Design review of the part built by this model. Coordinates are the model's own, in mm. A direction names the side the tool comes from. Give positions to 0.01 mm unless a question says otherwise; leave off trailing zeros. Order: outer loops, then holes, each group sorted by start corner. A loop starts at its lowest first (then second) coordinate and runs counter-clockwise, first axis right, second up.
```python
from build123d import *

# Parameters (mm, degrees)
ESQUISSE2_R                         = 1.35
BOSS_EXTRU_2_DEPTH                  = 6
BOSS_EXTRU_3_START                  = -6
ESQUISSE3_R                         = 1.35
BOSS_EXTRU_3_DEPTH                  = 6
ENL_V_MAT_EXTRU_1_REACH             = 49.73
ESQUISSE4_W                         = 8
ESQUISSE4_H                         = 4
ENL_V_MAT_EXTRU_1_DIRECTION_2_REACH = 49.73
CONG_1_R                            = 5


with BuildPart() as part:
    # Esquisse1 → Révolution1 (revolve)
    with BuildSketch(Plane.XY, mode=Mode.PRIVATE) as r_volution1_sk:
        Polygon((-6.05, 0), (-6.05, 4), (-3.85, 4), (-3.25, 4.6), (-3.25, 25.8), (-3.85, 26.4), (-6.05, 26.4), (-6.05, 30.4), (-8, 30.4), (-8, 24.4), (-5, 21.4), (-5, 9), (-8, 6), (-8, 0), align=None)
    revolve(r_volution1_sk.sketch.rotate(Axis((0, -1.144220684, 0), (0, 1, 0)), 270), axis=Axis((0, -1.144220684, 0), (0, 1, 0)))

    # Esquisse2 → Boss.-Extru.2 (add)
    with BuildSketch(Plane(origin=(0, 0, 0), x_dir=(1, 0, 0), z_dir=(0, 1, 0))):
        with BuildLine():
            Line((-7.878088106, -1.391304348), (-3.939044053, -23.695652174))
            ThreePointArc((-3.939044053, -23.695652174), (0, -27), (3.939044053, -23.695652174))
            Line((3.939044053, -23.695652174), (7.878088106, -1.391304348))
            ThreePointArc((7.878088106, -1.391304348), (0, -8), (-7.878088106, -1.391304348))
        make_face()
        with Locations(Location((0, -23, 0), (0, 0, 270))):
            Circle(ESQUISSE2_R, mode=Mode.SUBTRACT)
    extrude(amount=BOSS_EXTRU_2_DEPTH)

    # Esquisse3 → Boss.-Extru.3 (add)
    with BuildSketch(Plane(origin=(0, 30.4, 0), x_dir=(1, 0, 0), z_dir=(0, 1, 0)).offset(BOSS_EXTRU_3_START)):
        with BuildLine():
            Line((-21.761904762, -3.926767262), (-1.523809524, -7.853534525))
            ThreePointArc((-1.523809524, -7.853534525), (-8, 0), (-1.523809524, 7.853534525))
            Line((-1.523809524, 7.853534525), (-21.761904762, 3.926767262))
            ThreePointArc((-21.761904762, 3.926767262), (-25, 0), (-21.761904762, -3.926767262))
        make_face()
        with Locations(Location((-21, 0, 0), (0, 0, 270))):
            Circle(ESQUISSE3_R, mode=Mode.SUBTRACT)
    extrude(amount=BOSS_EXTRU_3_DEPTH)

    # Enlèv. mat.-Extru.1: up to this plane
    enl_v_mat_extru_1_end = Plane(origin=(-21.761904762, 24.4, -3.926767262), z_dir=(-0.19047619047618092, 0, -0.9816918156232545))
    # Esquisse4 → Enlèv. mat.-Extru.1 (cut, up to the surface)
    with BuildSketch(Plane.XY, mode=Mode.PRIVATE) as enl_v_mat_extru_1_sk1:
        with Locations((-21, 28.4)):
            Rectangle(ESQUISSE4_W, ESQUISSE4_H)
    enl_v_mat_extru_1_tool1 = split(extrude(enl_v_mat_extru_1_sk1.sketch, amount=-ENL_V_MAT_EXTRU_1_REACH, mode=Mode.PRIVATE), bisect_by=enl_v_mat_extru_1_end, keep=Keep.BOTH, mode=Mode.PRIVATE)
    add(enl_v_mat_extru_1_tool1.solids().sort_by_distance((-21, 28.4, 0))[0], mode=Mode.SUBTRACT)

    # Enlèv. mat.-Extru.1 direction 2: up to this plane
    enl_v_mat_extru_1_direction_2_end = Plane(origin=(-21.761904762, 24.4, 3.926767262), z_dir=(-0.19047619047620132, 0, 0.9816918156232504))
    # Esquisse4 → Enlèv. mat.-Extru.1 direction 2 (cut, up to the surface)
    with BuildSketch(Plane.XY, mode=Mode.PRIVATE) as enl_v_mat_extru_1_direction_2_sk1:
        with Locations((-21, 28.4)):
            Rectangle(ESQUISSE4_W, ESQUISSE4_H)
    enl_v_mat_extru_1_direction_2_tool1 = split(extrude(enl_v_mat_extru_1_direction_2_sk1.sketch, amount=ENL_V_MAT_EXTRU_1_DIRECTION_2_REACH, mode=Mode.PRIVATE), bisect_by=enl_v_mat_extru_1_direction_2_end, keep=Keep.BOTH, mode=Mode.PRIVATE)
    add(enl_v_mat_extru_1_direction_2_tool1.solids().sort_by_distance((-21, 28.4, 0))[0], mode=Mode.SUBTRACT)

    # Congé1
    cong_1_edges = [part.edges().sort_by_distance(p)[0] for p in [
        (-17, 28.4, -4.850712501),
        (-17, 28.4, 4.850712501),
    ]]
    fillet(cong_1_edges, radius=CONG_1_R)


solid = part.part
```
1. For line 1 along X through (y, z) = (25.7, 0); line 2 along X through (y, z) = (11, 0); line 3 along X through (y, z) = (2.05, 0), list the stretches that pass through material, from the lowest coordinate up.
Recorded:
line 1: x = -25 to -22.35, -19.65 to -3.25, 3.25 to 8
line 2: x = -5 to -3.25, 3.25 to 5
line 3: x = -8 to -6.05, 6.05 to 8
2. For pin 1 (3.5 mm diameter, centred on x = -21, z = 0, fed in from +Y); pin 2 (6 mm diameter, centred on x = -8.5, y = 19, fed in from +Z); pin 3 (1.6 mm diameter, centred on y = 28, z = 0, fed in from -X); pin 4 (6 mm diameter, centred on y = 6, z = 17.5, fed in from +X), all flat-tipped, find the tip position at first contact; note any pin that passes through.
Recorded:
pin 1: stops at y = 26.4
pin 2: passes through
pin 3: stops at x = -17
pin 4: stops at x = 5.56
3. Take a section at A-A (x = 0). State how many separate pieces and enclosed holes the cut face has, then the cut area to 3 significant figures.
Recorded:
separate pieces: 3
enclosed holes: 0
area: 249 mm2
4. Machinability: for faces 1 (the face through (-15.89, 28.43, -3.87)), 2 (the face through (-15.89, 28.43, 3.87)), 3 (the face through (1, 4, -4)), which of the approach directions +Z, -Z, +X, -X, +Y, -Y give a long, thin tool a straight path to every point of the face, cutting with its end or side? Answer none if there is none.
Recorded:
face 1: -Z, -X, +Y
face 2: +Z, -X, +Y
face 3: -Y
5. Take a section at D-D (x = -21). State the section outline as (y, z) points.
Recorded:
outline: (24.4, -4.07) - (26.4, -4.07) - (26.4, -1.35) - (24.4, -1.35) - close; (24.4, 1.35) - (26.4, 1.35) - (26.4, 4.07) - (24.4, 4.07) - close
6. Take a section at B-B (y = 25). State the section outline as (x, z) points.
Recorded:
outline: (-21.76, -3.93) - (-1.52, -7.85) arc R8 ccw (long way) to (-1.52, 7.85) - (-21.76, 3.93) arc R4 ccw to start; hole circle Ø2.7 at (-21, 0); hole circle Ø6.5 at (0, 0)
7. Draft analysis for pull direction Y (two halves, no side actions). For faces 4 (the face through (-1.82, 2.03, -5.77)), 5 (the face through (4.88, 15.11, 1.08)), 6 (the face through (-19, 26.4, 0)), state which applies: pulls with the +Y half, pulls with the -Y half, needs draft (parallel to the pull), parting line crosses it, or undercut.
Recorded:
face 4: needs draft
face 5: undercut
face 6: pulls with the +Y half
